Here's how the part is built. I have some questions about the finished solid (model axes, mm). A direction names the side the tool comes from. Coordinates: 2 decimals unless noted, no trailing zeros. Order: outer loops, then holes, each group sorted by start corner. A loop starts at its lowest first (then second) coordinate and runs counter-clockwise, first axis right, second up. Notation, with made-up numbers: (40, -6.75) - (47, -6.75) arc R9 cw to (47, 8.25) - close; hole circle Ø8 at (-30.5, 86). An arc over 180 degrees is marked (long way). Answer in a Markdown table with one row per item. Add a question column.
Item 1: I want a section at C-C (z = -2.25). Please give me the cut outline in (x, y).
Item 2: I want a section at D-D (x = 39). Please give me the cut outline in (y, z).
Item 3: Will these pins go through, and if not, where does the flat tip stop? pin 1 Ø5 at (x, y) = (90, 10) entering from -Z; pin 2 Ø3 at (x, y) = (81.5, 36) entering from +Z; pin 3 Ø2 at (x, y) = (54.5, 29) entering from +Z.
Item 4: I want a section at B-B (y = 50). Please give me the cut outline in (x, z), plus the area to 3 significant figures.
Item 5: Thinking about a two-plate mould opening in X: for faces 1 (the flat face through (0, 30, -15)), 2 (the flat face through (49, 10, 0)), 3 (the cylindrical face through (27.85, 18.01, -9.86)), which applies, +X half, -X half, draft (parallel to the pull), parting line (faces both ways), or undercut?
Item 6: I want a section at A-A (x = 90). Please give me the cut outline in (y, z), plus the area to 3 significant figures.
Item 7: On a 3-axis mill with a long thin cutter (end or side, diameter ignored), from which of +Z, -Z, +X, -X, +Y, -Y can I reach the whole of each face in a straight line? I mean faces 4 (the cylindrical face through (86, 10, -15)), 5 (the cylindrical face through (72.15, 41.99, -9.86)). Say none if no direction works.
Item 8: If I drill on line 1 along Y through (x, z) = (90, -8); line 2 along X through (y, z) = (13.5, -23.5); line 3 along Y through (x, z) = (8, -9.25), over which ranges is the centre line in solid material (lowest first)? Write a range as from..to.
```python
from build123d import *

# Parameters (mm, degrees)
ESBO_O1_W       = 100
ESBO_O1_H       = 60
ESBO_O1_R       = 4
EXTRUS_O2_DEPTH = 30
EXTRUS_O3_DEPTH = 20


with BuildPart() as part:
    # Esbo_o1 → Extrus_o2 (new body)
    with BuildSketch(Plane.XY):
        with Locations((50, 30)):
            Rectangle(ESBO_O1_W, ESBO_O1_H)
        with Locations((90, 10)):
            Circle(ESBO_O1_R, mode=Mode.SUBTRACT)
        with Locations((10, 10)):
            Circle(ESBO_O1_R, mode=Mode.SUBTRACT)
        with Locations((10, 50)):
            Circle(ESBO_O1_R, mode=Mode.SUBTRACT)
        with Locations((90, 50)):
            Circle(ESBO_O1_R, mode=Mode.SUBTRACT)
        with BuildLine():
            ThreePointArc((25, 25), (27.928932188, 17.928932188), (35, 15))
            Line((35, 15), (65, 15))
            ThreePointArc((65, 15), (72.071067812, 17.928932188), (75, 25))
            Line((75, 25), (75, 35))
            ThreePointArc((75, 35), (72.071067812, 42.071067812), (65, 45))
            Line((65, 45), (35, 45))
            ThreePointArc((35, 45), (27.928932188, 42.071067812), (25, 35))
            Line((25, 35), (25, 25))
        make_face(mode=Mode.SUBTRACT)
        with BuildLine():
            Line((25, 35), (25, 25))
            ThreePointArc((25, 25), (27.928932188, 17.928932188), (35, 15))
            Line((35, 15), (65, 15))
            ThreePointArc((65, 15), (72.071067812, 17.928932188), (75, 25))
            Line((75, 25), (75, 35))
            ThreePointArc((75, 35), (72.071067812, 42.071067812), (65, 45))
            Line((65, 45), (35, 45))
            ThreePointArc((35, 45), (27.928932188, 42.071067812), (25, 35))
        make_face()
    extrude(amount=-EXTRUS_O2_DEPTH)

    # Esbo_o1_4 → Extrus_o3 (cut)
    with BuildSketch(Plane.XY):
        with BuildLine():
            Line((25, 35), (25, 25))
            ThreePointArc((25, 25), (27.928932188, 17.928932188), (35, 15))
            Line((35, 15), (65, 15))
            ThreePointArc((65, 15), (72.071067812, 17.928932188), (75, 25))
            Line((75, 25), (75, 35))
            ThreePointArc((75, 35), (72.071067812, 42.071067812), (65, 45))
            Line((65, 45), (35, 45))
            ThreePointArc((35, 45), (27.928932188, 42.071067812), (25, 35))
        make_face()
    extrude(amount=-EXTRUS_O3_DEPTH, mode=Mode.SUBTRACT)


solid = part.part
```
Values follow:
| question | item | result |
|---|---|---|
| 1 | outline | (0, 0) - (100, 0) - (100, 60) - (0, 60) - close; hole circle Ø8 at (10, 10); hole circle Ø8 at (10, 50); hole (25, 25) arc R10 ccw to (35, 15) - (65, 15) arc R10 ccw to (75, 25) - (75, 35) arc R10 ccw to (65, 45) - (35, 45) arc R10 ccw to (25, 35) - close; hole circle Ø8 at (90, 10); hole circle Ø8 at (90, 50) |
| 2 | outline | (0, -30) - (60, -30) - (60, 0) - (45, 0) - (45, -20) - (15, -20) - (15, 0) - (0, 0) - close |
| 3 | pin 1 | passes through |
| 3 | pin 2 | stops at z = 0 |
| 3 | pin 3 | stops at z = -20 |
| 4 | outline | (0, -30) - (6, -30) - (6, 0) - (0, 0) - close; (14, -30) - (86, -30) - (86, 0) - (14, 0) - close; (94, -30) - (100, -30) - (100, 0) - (94, 0) - close |
| 4 | area | 2,520 mm^2 |
| 5 | face 1 | -X half |
| 5 | face 2 | draft |
| 5 | face 3 | undercut |
| 6 | outline | (0, -30) - (6, -30) - (6, 0) - (0, 0) - close; (14, -30) - (46, -30) - (46, 0) - (14, 0) - close; (54, -30) - (60, -30) - (60, 0) - (54, 0) - close |
| 6 | area | 1,320 mm^2 |
| 7 | face 4 | +Z, -Z |
| 7 | face 5 | +Z |
| 8 | line 1 | y = 0..6, 14..46, 54..60 |
| 8 | line 2 | x = 0..8.06, 11.94..88.06, 91.94..100 |
| 8 | line 3 | y = 0..6.54, 13.46..46.54, 53.46..60 |
